Geometry: final body of the model. Coordinates: model frame, mm. A direction names the side the tool comes from. Give positions to 0.01 mm unless a question says otherwise; leave off trailing zeros. Write each loop counter-clockwise with the first axis right and the second up, starting at its lowest first coordinate (ties: lowest second). Pieces come first, ordered by that corner, then holes. Notation, with made-up numbers: (-28, 1) -> (-5, 1) arc R10 ccw to (-5, 7) -> close; hole circle Ø9 at (88.5, 54.25). An arc over 180 degrees is marked (long way). Use CSV: the item, a comma, the result in double quotes. Start each with the question number.
1) Section C-C (x = 103.75). Output: boundary loops of the cut face in (y, z) (3 decimals), plus the area to 3 significant figures.
2) Section B-B (z = 38.75). Output: boundary loops of the cut face in (x, y) (3 decimals), plus the area to 3 significant figures.
3) Section D-D (z = 46). Output: boundary loops of the cut face in (x, y).
4) Material intervals for line 1 (Z direction, x = 107, y = -3.75); line 2 (Z direction, x = 103.75, y = 2) (3 decimals); line 3 (Y direction, x = 108.6, z = 46), sorted ascending. Write a range as [from, to].
5) Set-up query: faces 1 (the face through (110, -1, 32.5)), 2 (the face through (109.79, -2.42, 44.82)), 3 (the face through (32, 2, 27.35)). Return all of +Z, -Z, +X, -X, +Y, -Y with unobstructed straight access to the full face (end or side cutting, diameter ignored); none if empty.
6) Draft query along Z for faces 4 (the face through (112.75, -11, 20)), 5 (the face through (20.25, 2, 26)). Return one class per face: pulls with the +Z half, pulls with the -Z half, needs draft (parallel to the pull), parting line crosses it, or undercut.
7) Contact query for flat-ended pins moving along their axis: P1, Ø3, axis at x = 62, z = 11, coming from the -Y side; P2, Ø10, axis at x = 58, y = 3.5, coming from the -Z side; P3, Ø3.5, axis at x = 103.75, z = 38.75, coming from the +Y side; P4, Ø3, axis at y = -3.5, z = 46, coming from the -X side. Output: stop coordinate, or through.
8) Section A-A (y = 5.5). Output: boundary loops of the cut face in (x, z).
```python
from build123d import *

# Parameters (mm, degrees)
BOX011_W                   = 15
BOX011_H                   = 6
BOX011_DEPTH               = 4
EXTRUDE003_DEPTH           = 5
EXTRUDE003_ROLL_ANGLE      = -90
EXTRUDE003_PLACEMENT_ANGLE = -90
CYLINDER010_R              = 1.6
CYLINDER010_DEPTH          = 10
CYLINDER009_R              = 1.6
CYLINDER009_DEPTH          = 10
SKETCH_W                   = 106.75
SKETCH_H                   = 41.75
SKETCH_R                   = 1.625
EXTRUDE_DEPTH              = 8
EXTRUDE_PLACEMENT_ANGLE    = 270
BOX009_W                   = 6
BOX009_H                   = 17
BOX009_DEPTH               = 23
BOX005_W                   = 6
BOX005_H                   = 21
BOX005_DEPTH               = 64
TUBE003_R                  = 4
TUBE003_R_2                = 1.5
TUBE003_DEPTH              = 12


with BuildPart() as cube007:
    # Box011 → Box011 (new body)
    with BuildSketch(Plane(origin=(66.5, -0.9, 22.75), x_dir=(1, 0, 0), z_dir=(0, 0, 1))):
        with Locations((7.5, 3)):
            Rectangle(BOX011_W, BOX011_H)
    extrude(amount=BOX011_DEPTH)


with BuildPart() as extrude003:
    # Sketch004 → Extrude003 (new body)
    with BuildSketch(Plane.YZ):
        Polygon((10.25, 66.5), (10.25, 43.25), (12.9, 43.25), (12.9, 20.25), (16.15, 20.25), (16.15, 15.25), (24.15, 15.25), (24.15, 20.25), (27.4, 20.25), (27.4, 43.25), (30, 43.25), (30, 66.5), align=None)
    extrude(amount=EXTRUDE003_DEPTH)


with BuildPart() as extrude003_1:
    # Extrude003 roll: moved
    add(extrude003.part.rotate(Axis((0, 0, 0), (1, 0, 0)), EXTRUDE003_ROLL_ANGLE))


with BuildPart() as extrude003_2:
    # Extrude003 placement: moved
    add(extrude003_1.part.moved(Location((0, 4, 40.25))).rotate(Axis((0, 4, 40.25), (0, 0, 1)), EXTRUDE003_PLACEMENT_ANGLE))


with BuildPart() as cylinder010:
    # Cylinder010 → Cylinder010 (new body)
    with BuildSketch(Plane(origin=(114, 6.5, 46), x_dir=(0, 0, 1), z_dir=(-1, 0, 0))):
        Circle(CYLINDER010_R)
    extrude(amount=CYLINDER010_DEPTH)


with BuildPart() as m3cyl:
    # Cylinder009 → Cylinder009 (new body)
    with BuildSketch(Plane(origin=(114, 6.5, -6), x_dir=(0, 0, 1), z_dir=(-1, 0, 0))):
        Circle(CYLINDER009_R)
    extrude(amount=CYLINDER009_DEPTH)

    # Fusion010: union Cylinder010
    add(cylinder010.part)


with BuildPart() as m3cyl_1:
    # Fusion010 placement: moved
    add(m3cyl.part.moved(Location((0, -10, 0))))


with BuildPart() as bottom:
    # Sketch → Extrude (new body)
    with BuildSketch(Plane.YZ):
        with Locations((53.375, 20.875)):
            Rectangle(SKETCH_W, SKETCH_H)
        with Locations((3, 3)):
            Circle(SKETCH_R, mode=Mode.SUBTRACT)
        with Locations((3, 38.75)):
            Circle(SKETCH_R, mode=Mode.SUBTRACT)
        with Locations((103.75, 38.75)):
            Circle(SKETCH_R, mode=Mode.SUBTRACT)
        with Locations((103.75, 3)):
            Circle(SKETCH_R, mode=Mode.SUBTRACT)
    extrude(amount=EXTRUDE_DEPTH)


with BuildPart() as bottom_1:
    # Extrude placement: moved
    add(bottom.part.moved(Location((0, 4, 0))).rotate(Axis((0, 4, 0), (0, 0, 1)), EXTRUDE_PLACEMENT_ANGLE))


with BuildPart() as basemount001:
    # Box009 → Box009 (new body)
    with BuildSketch(Plane(origin=(106.75, 0, 9.5), x_dir=(1, 0, 0), z_dir=(0, 0, 1))):
        with Locations((3, 8.5)):
            Rectangle(BOX009_W, BOX009_H)
    extrude(amount=BOX009_DEPTH)


with BuildPart() as obj1:
    # Box005 → Box005 (new body)
    with BuildSketch(Plane(origin=(106.75, -4, -12), x_dir=(1, 0, 0), z_dir=(0, 0, 1))):
        with Locations((3, 10.5)):
            Rectangle(BOX005_W, BOX005_H)
    extrude(amount=BOX005_DEPTH)

    # Cut001: cut baseMOunt001
    add(basemount001.part, mode=Mode.SUBTRACT)


with BuildPart() as obj1_1:
    # Cut001 placement: moved
    add(obj1.part.moved(Location((0, -10, 0))))

    # Fusion009: union Bottom
    add(bottom_1.part)

    # Cut002: cut m3Cyl
    add(m3cyl_1.part, mode=Mode.SUBTRACT)

    # Cut003: cut Extrude003
    add(extrude003_2.part, mode=Mode.SUBTRACT)

    # Cut004: cut Cube007
    add(cube007.part, mode=Mode.SUBTRACT)


with BuildPart() as bottom001:
    # Tube003 → Tube003 (new body)
    with BuildSketch(Plane(origin=(71, 12, 18.5), x_dir=(0, 0, -1), z_dir=(0, -1, 0))):
        Circle(TUBE003_R)
        Circle(TUBE003_R_2, mode=Mode.SUBTRACT)
    extrude(amount=TUBE003_DEPTH)

    # Fusion011: union obj1
    add(obj1_1.part)


solid = bottom001.part
```
Answers follow:
1,outline,"(-4, 0) -> (4, 0) -> (4, 1.375) -> (-4, 1.375) -> close; (-4, 4.625) -> (4, 4.625) -> (4, 37.125) -> (-4, 37.125) -> close; (-4, 40.375) -> (4, 40.375) -> (4, 41.75) -> (-4, 41.75) -> close"
1,area,"282 mm^2"
2,outline,"(0, -4) -> (1.375, -4) -> (1.375, 4) -> (0, 4) -> close; (4.625, -4) -> (102.125, -4) -> (102.125, 4) -> (4.625, 4) -> close; (105.375, -4) -> (106.75, -4) -> (106.75, -14) -> (112.75, -14) -> (112.75, 7) -> (106.75, 7) -> (106.75, 4) -> (105.375, 4) -> close"
2,area,"928 mm^2"
3,outline,"(106.75, -14) -> (112.75, -14) -> (112.75, -5.1) -> (106.75, -5.1) -> close; (106.75, -1.9) -> (112.75, -1.9) -> (112.75, 7) -> (106.75, 7) -> close"
4,line 1,"z = [-12, -7.58], [-4.42, 9.5], [32.5, 44.42], [47.58, 52]"
4,line 2,"z = [0, 1.375], [4.625, 37.125], [40.375, 41.75]"
4,line 3,"y = [-14, -5.1], [-1.9, 7]"
5,face 1,"+X, +Y"
5,face 2,"+X, -X"
5,face 3,"+Y"
6,face 4,"needs draft"
6,face 5,"undercut"
7,P1,"stops at y = -4"
7,P2,"stops at z = 0"
7,P3,"stops at y = 4"
7,P4,"passes through"
8,outline,"circle Ø8 at (71, 18.5); (106.75, -12) -> (112.75, -12) -> (112.75, 9.5) -> (106.75, 9.5) -> close; (106.75, 32.5) -> (112.75, 32.5) -> (112.75, 52) -> (106.75, 52) -> close; hole circle Ø3 at (71, 18.5)"
